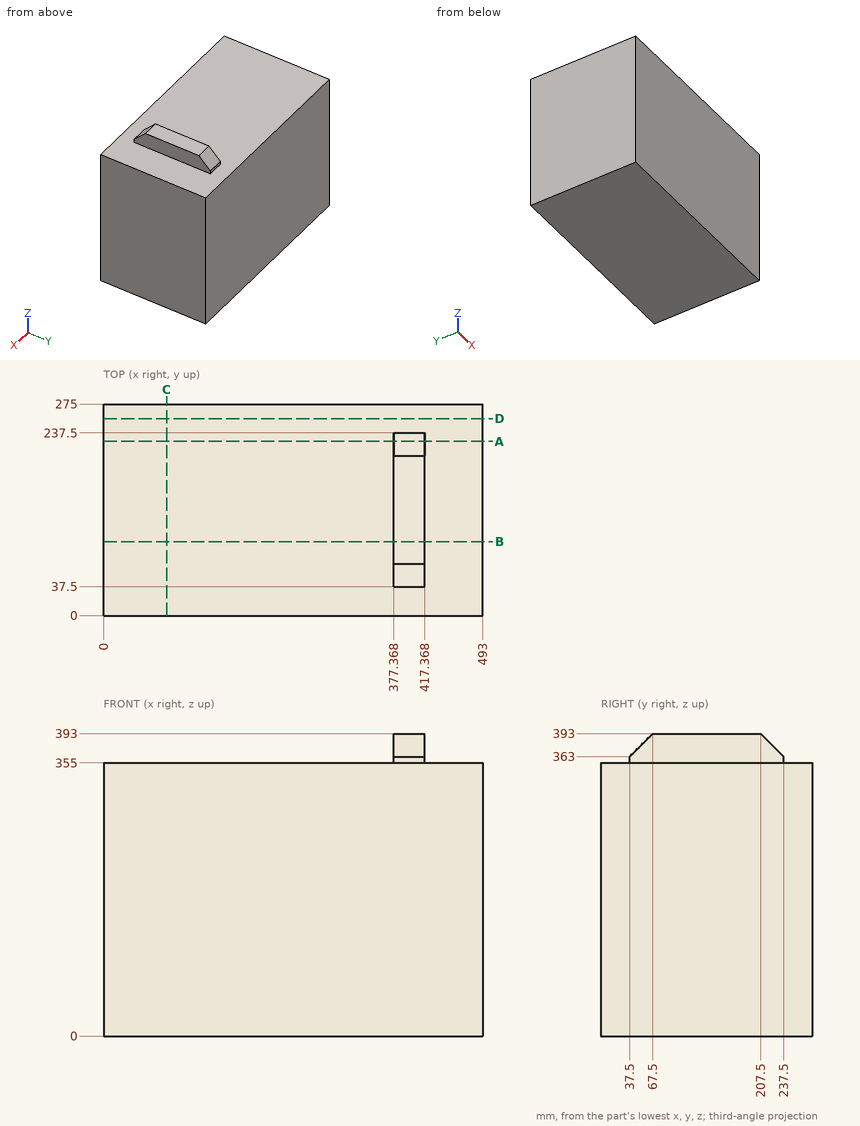
Input: dimensioned drawing with shaded views. Units: mm. Origin: part minimum x, y, z. Give positions to 0.01 mm unless a question says otherwise; leave off trailing zeros. Write each loop counter-clockwise with the first axis right and the second up, starting at its lowest first coordinate (ties: lowest second). Pieces come first, ordered by that corner, then holes. Notation, with made-up numbers: (-31, 31) -> (14, 31) arc R20 cw to (14, 66) -> close; hole circle Ø10 at (88, 74). An arc over 180 degrees is marked (long way). Return JSON: item names as keys, results as strings. Group by question number.
1. Material intervals for line 1 (Z direction, x = 30, y = 73); line 2 (X direction, y = 179.5, z = 372.5), sorted ascending. Write a range as from..to.
2. Section D-D, the plane y = 256. Output: boundary loops of the cut face in (x, z).
3. Section B-B, the plane y = 96. Output: boundary loops of the cut face in (x, z), then the cut area to 3 significant figures.
4. Pin query (flat end, axial travel): pin 1 Ø2 at (x, y) = (173, 40) entering from +Z; pin 2 Ø6.5 at (x, z) = (401.5, 360.5) entering from +Y; pin 3 Ø11.5 at (y, z) = (94.5, 379.5) entering from +X. Return the tip coordinate at first contact, or that it passes through.
5. Section C-C, the plane x = 82. Output: boundary loops of the cut face in (y, z).
6. Section A-A, the plane y = 226.5. Output: boundary loops of the cut face in (x, z).
Determined:
{
 "1": {"line 1": "z = 0..355", "line 2": "x = 377.37..417.37"},
 "2": {"outline": "(0, 0) -> (493, 0) -> (493, 355) -> (0, 355) -> close"},
 "3": {"outline": "(0, 0) -> (493, 0) -> (493, 355) -> (417.37, 355) -> (417.37, 393) -> (377.37, 393) -> (377.37, 355) -> (0, 355) -> close", "area": "177,000 mm2"},
 "4": {"pin 1": "stops at z = 355", "pin 2": "stops at y = 237.5", "pin 3": "stops at x = 417.37"},
 "5": {"outline": "(0, 0) -> (275, 0) -> (275, 355) -> (0, 355) -> close"},
 "6": {"outline": "(0, 0) -> (493, 0) -> (493, 355) -> (417.37, 355) -> (417.37, 374) -> (377.37, 374) -> (377.37, 355) -> (0, 355) -> close"}
}
